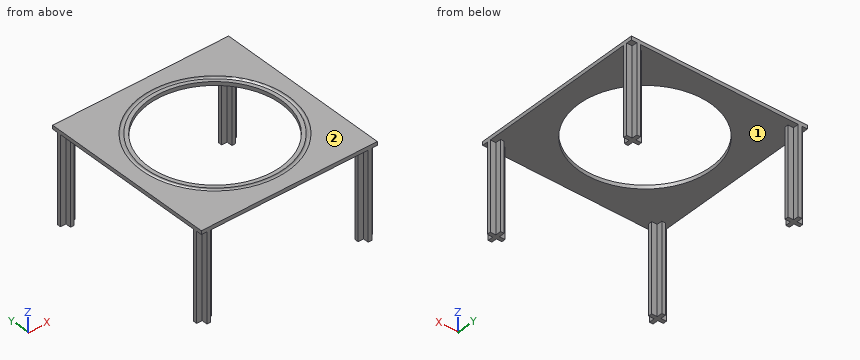
```python
from build123d import *

# Parameters (mm, degrees)
F0_W     = 609.6
F0_H     = 609.6
F1_DEPTH = 6.35
F3_DEPTH = 304.8
F4_R     = 228.6
F8_DEPTH = 317.501


with BuildPart() as f1:
    # F0 (on Top) → F1 (new body, symmetric)
    with BuildSketch(Plane.XY):
        with Locations((304.8, 304.8)):
            Rectangle(F0_W, F0_H)
    extrude(amount=F1_DEPTH, both=True)

    # F2 (on face) → F3 (join)
    with BuildSketch(Plane(origin=(0, 0, -6.35), x_dir=(1, 0, 0), z_dir=(0, 0, -1))):
        Polygon((19.05, -19.05), (0, -19.05), (0, -31.75), (19.05, -31.75), (19.05, -50.8), (31.75, -50.8), (31.75, -31.75), (50.8, -31.75), (50.8, -19.05), (31.75, -19.05), (31.75, 0), (19.05, 0), align=None)
        Polygon((590.55, -50.8), (590.55, -31.75), (609.6, -31.75), (609.6, -19.05), (590.55, -19.05), (590.55, 0), (577.85, 0), (577.85, -19.05), (558.8, -19.05), (558.8, -31.75), (577.85, -31.75), (577.85, -50.8), align=None)
        Polygon((19.05, -590.55), (19.05, -609.6), (31.75, -609.6), (31.75, -590.55), (50.8, -590.55), (50.8, -577.85), (31.75, -577.85), (31.75, -558.8), (19.05, -558.8), (19.05, -577.85), (0, -577.85), (0, -590.55), align=None)
        Polygon((577.85, -609.6), (590.55, -609.6), (590.55, -590.55), (609.6, -590.55), (609.6, -577.85), (590.55, -577.85), (590.55, -558.8), (577.85, -558.8), (577.85, -577.85), (558.8, -577.85), (558.8, -590.55), (577.85, -590.55), align=None)
    extrude(amount=F3_DEPTH)

    # F6 (on offset) → F7 (revolve, cut)
    with BuildSketch(Plane.XZ.offset(-304.8)):
        with BuildLine():
            Line((63.5, 6.35), (50.8, 6.35))
            ThreePointArc((50.8, 6.35), (57.15, -0.1598234894), (63.5, 6.35))
        make_face()
    revolve(axis=Axis((304.8, 304.8, 0), (0, 0, -1)), mode=Mode.SUBTRACT)

    # F4 (on face) → F8 (cut, through all)
    with BuildSketch(Plane.XY.offset(6.35)):
        with Locations((304.8, 304.8)):
            Circle(F4_R)
    extrude(amount=-F8_DEPTH, mode=Mode.SUBTRACT)


solid = f1.part
```
Can you work these out from the model? Positions are in its coordinate system, mm. Face numbers are marked on the shaded views. Give positions to 0.01 mm unless a question says otherwise; leave off trailing zeros. Order: outer loops, then holes, each group sorted by start corner. A loop starts at its lowest first (then second) coordinate and runs counter-clockwise, first axis right, second up. Notation, with made-up numbers: M 68,-12 L 95,-12 A16 cw 95,7 Z; hole C 88,41 d10. An arc over 180 degrees is marked long. Write item = value, one per line. Start each with the question number.
Q1. Suppose I cut it at C-C (z = -276). Count the separate pieces of the cut face and the enclosed holes in it, plus the area to 3 significant figures.
Q2. Suppose I cut it at A-A (y = 304.8). Write out the boundary of the cut face in (x, z).
Q3. We'd pull the mould along Y, two halves only. Please class the marked faces 1 and 2: pulls with the +Y half, pulls with the -Y half, needs draft (parallel to the pull), parting line crosses it, or undercut.
Q4. I need wall thicknesses on probe 1 along Y at (x, z) = (304.8, -2); probe 2 along X at (y, z) = (48.5, -234); probe 3 along Y at (x, z) = (304.8, 2.25). Which ranges of each line are inside material? Lowest first, please. Write a range as [from, to].
Q5. Will these pins go through, and if not, where does the flat tip stop? pin 1 Ø5.5 at (x, z) = (5.5, -163) entering from +Y; pin 2 Ø15 at (y, z) = (572.5, -201) entering from +X; pin 3 Ø21 at (y, z) = (602.5, -225.5) entering from +X; pin 4 Ø21 at (x, y) = (602.5, 6) entering from -Z.
Check result:
q1.separate_pieces = 4
q1.enclosed_holes = 0
q1.area = 4,520 mm2
q2.outline = M 0,-6.35 L 76.2,-6.35 L 76.2,6.35 L 63.5,6.35 A6.35 cw long 50.8,6.35 L 0,6.35 Z; M 533.4,-6.35 L 609.6,-6.35 L 609.6,6.35 L 558.8,6.35 A6.35 cw long 546.1,6.35 L 533.4,6.35 Z
q3.face_1 = undercut
q3.face_2 = needs draft
q4.probe_1 = [0, 76.2], [533.4, 609.6]
q4.probe_2 = [19.05, 31.75], [577.85, 590.55]
q4.probe_3 = [0, 52.17], [62.13, 76.2], [533.4, 547.47], [557.43, 609.6]
q5.pin_1 = 590.55
q5.pin_2 = 609.6
q5.pin_3 = 590.55
q5.pin_4 = -6.35
